```python
from build123d import *

# Parameters (mm, degrees)
F2_SIZE  = 1
F4_DEPTH = 20


with BuildPart() as f1:
    # F0 (on Front) → F1 (revolve)
    with BuildSketch(Plane.XZ):
        Polygon((0, 10), (0, 0), (20, 0), (20, 17), (10, 17), (10, 10), align=None)
    revolve(axis=Axis((10, 0, 0), (1, 0, 0)))

    # F2
    f2_edges = [f1.edges().sort_by_distance(p)[0] for p in [
        (10, 0, -17),
        (0, 0, -10),
        (20, 0, -17),
    ]]
    chamfer(f2_edges, length=F2_SIZE)

    # F3 (on face) → F4 (cut)
    with BuildSketch(Plane.YZ.offset(20)):
        with BuildLine():
            Line((-1.5, 6.8), (-1.5, 4.769696))
            ThreePointArc((-1.5, 4.769696), (0, -5), (1.5, 4.769696))
            Line((1.5, 4.769696), (1.5, 6.8))
            Line((1.5, 6.8), (0, 6.8))
            Line((0, 6.8), (-1.5, 6.8))
        make_face()
    extrude(amount=-F4_DEPTH, mode=Mode.SUBTRACT)


solid = f1.part
```
For this review, take the finished solid that the model builds, in its own axes (mm). A direction names the side the tool comes from. Round coordinates to 2 decimals unless told otherwise and drop trailing zeros. Write each loop counter-clockwise with the first axis right and the second up, starting at its lowest first coordinate (ties: lowest second). Pieces come first, ordered by that corner, then holes. Notation, with made-up numbers: M 55,21 L 86,21 A19 ccw 86,48 Z; hole C -15.75,28.25 d9. An arc over 180 degrees is marked long. One line per item, written item: value. Start each with the question number.
(1) We need section C-C (x = 9). Give the boundary of the cut face in (y, z), and give its area (3 significant figures).
(2) We need section B-B (z = 0). Give the boundary of the cut face in (x, y).
(3) Machinability: for faces 1 (the flat face through (0, 4, 4)), 2 (the flat face through (10, 1.5, 6)), 3 (the flat face through (10, 10.4, -0.2)), which of the approach directions +Z, -Z, +X, -X, +Y, -Y give a long, thin tool a straight path to every point of the face, cutting with its end or side? Answer none if there is none.
(4) The part is to be moulded in two halves that separate along Y. For faces 4 (the cylindrical face through (5.44, 9.76, -2.17)), 5 (the flat face through (10, -1.5, 6)), 6 (the flat face through (20, -4, 4)), say which applies: released by +Y, released by -Y, zero draft, split by the parting line, or undercut.
(5) Wall thickness on line 1 (Y direction, x = 12.75, z = 0); line 2 (Z direction, x = 12.5, y = 0); line 3 (Y direction, x = 5.25, z = 0): over which ranges is each line inside the solid? List them lowest first.
(6) Insertion check: pin 1 (10 mm diameter, centred on x = 8, y = -11, fed in from +Z); pin 2 (1 mm diameter, centred on x = 7, z = 5.5, fed in from +Y); pin 3 (4 mm diameter, centred on x = 15.5, z = 13, fed in from -Y). Each pin has a flat end and moves straight along its axis. Give the tip position at first contact, or say it passes through.
(7) We need section A-A (y = 0). Give the boundary of the cut face in (x, z), and give its area (3 significant figures).
Result:
1. outline: C 0,0 d20; hole M -1.5,4.77 A5 ccw long 1.5,4.77 L 1.5,6.8 L -1.5,6.8 Z
1. area: 230 mm²
2. outline: M 0,-9 L 1,-10 L 10,-10 L 10,-16 L 11,-17 L 19,-17 L 20,-16 L 20,-5 L 0,-5 Z; M 0,5 L 20,5 L 20,16 L 19,17 L 11,17 L 10,16 L 10,10 L 1,10 L 0,9 Z
3. face 1: +Z, -Z, -X, +Y, -Y
3. face 2: +X, -X
3. face 3: -X
4. face 4: split by the parting line
4. face 5: undercut
4. face 6: zero draft
5. line 1: -17 to -5, 5 to 17
5. line 2: -17 to -5, 6.8 to 17
5. line 3: -10 to -5, 5 to 10
6. pin 1: z = 15.49
6. pin 2: y = 8.66
6. pin 3: y = -12.96
7. outline: M 0,-9 L 1,-10 L 10,-10 L 10,-16 L 11,-17 L 19,-17 L 20,-16 L 20,-5 L 0,-5 Z; M 0,6.8 L 20,6.8 L 20,16 L 19,17 L 11,17 L 10,16 L 10,10 L 1,10 L 0,9 Z
7. area: 301 mm²
